Check sheet for the modelled part. Datum: model origin and axes. Units: mm. A direction names the side the tool comes from. Round coordinates to 2 decimals unless told otherwise and drop trailing zeros. Write each loop counter-clockwise with the first axis right and the second up, starting at its lowest first coordinate (ties: lowest second). Pieces come first, ordered by that corner, then holes.
Item 1: Material ranges on line 1 (Z direction, x = 16, y = -6.5); line 2 (X direction, y = 15.5, z = -15); line 3 (X direction, y = -2, z = -4), recorded low to high.
Item 2: Cross-section at C-C on z = -24. Enter the section's corners in (x, y).
Item 3: Cross-section at A-A on y = 0. Enter the section's corners in (x, z), plus the area to 3 significant figures.
Item 4: Go/stop test with flat-tipped pins: pin 1 Ø6 at (x, z) = (12, -19) entering from +Y; pin 2 Ø8 at (y, z) = (5, -7.5) entering from -X; pin 3 Ø4 at (y, z) = (13.5, -7) entering from +X. Record where each tip stops, or that it passes through.
Item 5: Tool access check on faces 1 (the flat face through (0, 0, -35)), 2 (the cylindrical face through (-14.985, 0.66, 7.395)), 3 (the flat face through (-11, 11, -20)). Record the directions out of +Z, -Z, +X, -X, +Y, -Y that give a thin tool (end or side, any length) a straight path to the whole face; none if there is none.
Item 6: Cross-section at D-D on z = -9.5. Enter the section's corners in (x, y), plus the area to 3 significant figures.
from build123d import *

# Parameters (mm, degrees)
F0_R     = 15
F1_DEPTH = 15
F2_R     = 20.49161
F3_DEPTH = 20
F4_R     = 15
F5_DEPTH = 35


with BuildPart() as f1:
    # F0 (on Top) → F1 (new body)
    with BuildSketch(Plane.XY):
        Circle(F0_R)
    extrude(amount=F1_DEPTH)

    # F2 (on Top) → F3 (join)
    with BuildSketch(Plane.XY):
        Circle(F2_R)
    extrude(amount=-F3_DEPTH)

    # F4 (on Top) → F5 (join)
    with BuildSketch(Plane.XY):
        Circle(F4_R)
    extrude(amount=-F5_DEPTH)


solid = f1.part
Response values:
1. line 1: z = -20 to 0
1. line 2: x = -13.4 to 13.4
1. line 3: x = -20.39 to 20.39
2. outline: circle Ø30 at (0, 0)
3. outline: (-20.49, -20) - (-15, -20) - (-15, -35) - (15, -35) - (15, -20) - (20.49, -20) - (20.49, 0) - (15, 0) - (15, 15) - (-15, 15) - (-15, 0) - (-20.49, 0) - close
3. area: 1,720 mm2
4. pin 1: stops at y = 18.41
4. pin 2: stops at x = -20.47
4. pin 3: stops at x = 16.96
5. face 1: -Z, +X, -X, +Y, -Y
5. face 2: +Z
5. face 3: -Z
6. outline: circle Ø40.98 at (0, 0)
6. area: 1,320 mm2
